Here's how the part is built. I have some questions about the finished solid (model axes, mm). A direction names the side the tool comes from. Coordinates: 2 decimals unless noted, no trailing zeros. Write each loop counter-clockwise with the first axis right and the second up, starting at its lowest first coordinate (ties: lowest second). Pieces come first, ordered by that corner, then holes. Notation, with made-up numbers: (21, 15) -> (43, 15) arc R21 ccw to (43, 46) -> close; hole circle Ø3 at (-19, -25). An arc over 180 degrees is marked (long way). Answer in a Markdown table with one row per item. Add a question column.
from build123d import *

# Parameters (mm, degrees)
F1_R = 13.97
F3_R = 10.795


with BuildPart() as f2:
    # F2: sweep along a path in F0
    with BuildLine(Plane.XZ) as f2_path:
        Line((0, 0), (0, 21.14))
        ThreePointArc((0, 21.14), (6.6955389821, 37.3044610179), (22.86, 44))
        Line((22.86, 44), (44, 44))
    # F1 (on Top) → F2 (sweep)
    with BuildSketch(Plane.XY):
        Circle(F1_R)
    sweep(path=f2_path.line)

    # F4: sweep along a path in F0
    with BuildLine(Plane.XZ) as f4_path:
        Line((0, 0), (0, 21.14))
        ThreePointArc((0, 21.14), (6.6955389821, 37.3044610179), (22.86, 44))
        Line((22.86, 44), (44, 44))
    # F3 (on face) → F4 (sweep, cut)
    with BuildSketch(Plane(origin=(0, 0, 0), x_dir=(1, 0, 0), z_dir=(0, 0, -1))):
        Circle(F3_R)
    sweep(path=f4_path.line, mode=Mode.SUBTRACT)


solid = f2.part
Q1. For faces 5 (the flat face through (44, 10.3, 48.1)), 6 (the cylindrical face through (33.578, 4.196, 30.675)), which set-ups out of +Z, -Z, +X, -X, +Y, -Y let a thin tool reach every point of the face, with its end or its side?
Q2. Imagine slicing it at A-A on y = 0. Please give me the cut outline in (x, z) (3 decimals).
Q3. If we mould it in two halves opening along Y, with no side actions, what happens to faces 1 (the cylindrical face through (-7.956, 7.296, 10.718)), 2 (the cylindrical face through (33.578, 0.475, 54.785)), 3 (the flat face through (4.1, -10.3, 0)), 4 (the cylindrical face through (-1.82, 13.85, 10.72))? For each: pulls with the +Y half, pulls with the -Y half, needs draft (parallel to the pull), parting line crosses it, or undercut.
Q4. I'm going to push flat-ended pins straight in: P1, Ø10, axis at y = -1.5, z = 22.5, coming from the +X side; P2, Ø6, axis at y = 10.5, z = 29, coming from the +X side; P3, Ø1.5, axis at y = -10.5, z = 11, coming from the -X side. Where does each tip first touch, or does it pass through?
Q5. Imagine slicing it at B-B on x = 26. Please give me the cut outline in (y, z) (3 decimals).
Q6. Imagine slicing it at D-D on y = -4. Please give me the cut outline in (x, z), plus the area to 3 significant figures.
Q7. I need wall thicknesses on line 1 (Y direction, x = 33.5, z = 44) (3 decimals); line 2 (Y direction, x = 3.5, z = 12); line 3 (X direction, y = -1, z = 21.5). Which ranges of each line are inside material? Lowest first, please. Write a range as [from, to].
Q8. Imagine slicing it at C-C on z = 10.5. Please give me the cut outline in (x, y) (3 decimals), plus the area to 3 significant figures.
Result sheet:
| question | item | result |
|---|---|---|
| 1 | face 5 | +Z, -Z, +X, +Y, -Y |
| 1 | face 6 | +X |
| 2 | outline | (-13.97, 0) -> (-10.795, 0) -> (-10.795, 21.14) arc R33.655 cw to (22.86, 54.795) -> (44, 54.795) -> (44, 57.97) -> (22.86, 57.97) arc R36.83 ccw to (-13.97, 21.14) -> close; (10.795, 0) -> (13.97, 0) -> (13.97, 21.14) arc R8.89 cw to (22.86, 30.03) -> (44, 30.03) -> (44, 33.205) -> (22.86, 33.205) arc R12.065 ccw to (10.795, 21.14) -> close |
| 3 | face 1 | undercut |
| 3 | face 2 | undercut |
| 3 | face 3 | needs draft |
| 3 | face 4 | parting line crosses it |
| 4 | P1 | stops at x = 16.57 |
| 4 | P2 | stops at x = 16.8 |
| 4 | P3 | stops at x = -10 |
| 5 | outline | circle Ø27.94 at (0, 44); hole circle Ø21.59 at (0, 44) |
| 6 | outline | (-13.39, 0) -> (-10.03, 0) -> (-10.03, 21.14) arc R32.89 cw to (22.86, 54.03) -> (44, 54.03) -> (44, 57.39) -> (22.86, 57.39) arc R36.25 ccw to (-13.39, 21.14) -> close; (10.03, 0) -> (13.39, 0) -> (13.39, 21.14) arc R9.47 cw to (22.86, 30.61) -> (44, 30.61) -> (44, 33.97) -> (22.86, 33.97) arc R12.83 ccw to (10.03, 21.14) -> close |
| 6 | area | 525 mm^2 |
| 7 | line 1 | y = [-13.97, -10.795], [10.795, 13.97] |
| 7 | line 2 | y = [-13.52, -10.21], [10.21, 13.52] |
| 7 | line 3 | x = [-13.93, -10.75], [10.75, 13.94] |
| 8 | outline | circle Ø27.94 at (0, 0); hole circle Ø21.59 at (0, 0) |
| 8 | area | 247 mm^2 |
